```python
from build123d import *

# Parameters (mm, degrees)
SKETCH1_W           = 70
SKETCH1_H           = 70
BOSS_EXTRUDE1_DEPTH = 2
SKETCH2_W           = 50
SKETCH2_H           = 50
BOSS_EXTRUDE2_DEPTH = 35
SKETCH3_R           = 11
CUT_EXTRUDE1_DEPTH  = 6
SKETCH4_R           = 10
CUT_EXTRUDE2_DEPTH  = 2
SKETCH5_W           = 26.5
SKETCH5_H           = 12.5
CUT_EXTRUDE3_DEPTH  = 106.683489723
SKETCH7_W           = 5
SKETCH7_H           = 5.02305645
CUT_EXTRUDE4_DEPTH  = 96.557574268
SKETCH8_W           = 5
SKETCH8_H           = 12.5
CUT_EXTRUDE5_DEPTH  = 18


with BuildPart() as part:
    # Sketch1 → Boss-Extrude1 (new body)
    with BuildSketch(Plane.XY):
        with Locations((35, -35)):
            Rectangle(SKETCH1_W, SKETCH1_H)
    extrude(amount=BOSS_EXTRUDE1_DEPTH)

    # Sketch2 → Boss-Extrude2 (add)
    with BuildSketch(Plane.XY.offset(2)):
        with Locations((35, -35)):
            Rectangle(SKETCH2_W, SKETCH2_H)
    extrude(amount=BOSS_EXTRUDE2_DEPTH)

    # Sketch3 → Cut-Extrude1 (cut)
    with BuildSketch(Plane.XY.offset(37)):
        with Locations((35, -35)):
            Circle(SKETCH3_R)
    extrude(amount=-CUT_EXTRUDE1_DEPTH, mode=Mode.SUBTRACT)

    # Sketch4 → Cut-Extrude2 (cut)
    with BuildSketch(Plane.XY.offset(31)):
        with Locations((35, -35)):
            Circle(SKETCH4_R)
    extrude(amount=-CUT_EXTRUDE2_DEPTH, mode=Mode.SUBTRACT)

    # Sketch5 → Cut-Extrude3 (cut, through all)
    with BuildSketch(Plane.XY.offset(37)):
        with Locations((40.25, -35)):
            Rectangle(SKETCH5_W, SKETCH5_H)
    extrude(amount=-CUT_EXTRUDE3_DEPTH, mode=Mode.SUBTRACT)

    # Sketch7 → Cut-Extrude4 (cut, through all)
    with BuildSketch(Plane.ZY.offset(-53.5)):
        with Locations((2.5, -35)):
            Rectangle(SKETCH7_W, SKETCH7_H)
    extrude(amount=CUT_EXTRUDE4_DEPTH, mode=Mode.SUBTRACT)

    # Sketch8 → Cut-Extrude5 (cut)
    with BuildSketch(Plane.XY.offset(37)):
        with Locations((56, -35)):
            Rectangle(SKETCH8_W, SKETCH8_H)
        with Locations((24.5, -35)):
            Rectangle(SKETCH8_W, SKETCH8_H)
    extrude(amount=-CUT_EXTRUDE5_DEPTH, mode=Mode.SUBTRACT)


solid = part.part
```
Source: CAD feature listing. Evaluate the final solid. Frame: model axes, mm. A direction names the side the tool comes from. Coordinates: 2 decimals unless noted, no trailing zeros. Write each loop counter-clockwise with the first axis right and the second up, starting at its lowest first coordinate (ties: lowest second). Pieces come first, ordered by that corner, then holes. Notation, with made-up numbers: (42, 68) -> (88, 68) arc R22 cw to (88, 74) -> close; hole circle Ø11 at (-22, 9.25). An arc over 180 degrees is marked (long way). Return JSON: item names as keys, results as strings. Group by question number.
1) Section query A-A, the plane y = -35.5. Return loops of the section in (x, z).
2) Section query C-C, the plane x = 11.5. Return loops of the section in (y, z), plus the area to 3 significant figures.
3) Set-up query: faces 1 (the face through (60, -35, 19)), 2 (the face through (35, -60, 19)), 3 (the face through (35, -10, 19)), 4 (the face through (35, -45.2, 31)). Return all of +Z, -Z, +X, -X, +Y, -Y with unobstructed straight access to the full face (end or side cutting, diameter ignored); none if empty.
4) Section query B-B, the plane z = 14. Return loops of the section in (x, y), plus the area to 3 significant figures.
5) Ray query, line 1 along X through (y, z) = (-32, 8); line 2 along Y through (x, z) = (48.5, 3.5); line 3 along X through (y, z) = (-29.5, 28). Return the intervals inside material, ascending.
6) Mould query, pull axis X, two halves, no side actions, for faces 5 (the face through (24, -35, 19)), 6 (the face through (10, -35, 19)), 7 (the face through (66, -35, 2)). Classes: +X half, -X half, draft (parallel to the pull), parting line (faces both ways), or undercut.
7) Section query D-D, the plane y = -56. Return loops of the section in (x, z).
8) Contact query for flat-ended pins moving along their axis: P1, Ø2.5, axis at x = 34, y = -26.5, coming from the +Z side; P2, Ø5.5, axis at x = 56.5, y = -35.5, coming from the +Z side; P3, Ø2, axis at x = 44, z = 8, coming from the +Y side; P4, Ø17.5, axis at y = -30.5, z = 15.5, coming from the -X side. Output: stop coordinate, or through.
From the geometry:
{
 "1": {"outline": "(10, 5) -> (27, 5) -> (27, 19) -> (22, 19) -> (22, 37) -> (10, 37) -> close; (53.5, 0) -> (70, 0) -> (70, 2) -> (60, 2) -> (60, 37) -> (58.5, 37) -> (58.5, 19) -> (53.5, 19) -> close"},
 "2": {"outline": "(-70, 0) -> (-37.51, 0) -> (-37.51, 5) -> (-32.49, 5) -> (-32.49, 0) -> (0, 0) -> (0, 2) -> (-10, 2) -> (-10, 37) -> (-60, 37) -> (-60, 2) -> (-70, 2) -> close", "area": "1,860 mm²"},
 "3": {"face 1": "+Z, +X, +Y, -Y", "face 2": "+Z, +X, -X, -Y", "face 3": "+Z, +X, -X, +Y", "face 4": "+Z"},
 "4": {"outline": "(10, -60) -> (60, -60) -> (60, -10) -> (10, -10) -> close; hole (27, -41.25) -> (53.5, -41.25) -> (53.5, -28.75) -> (27, -28.75) -> close", "area": "2,170 mm²"},
 "5": {"line 1": "10 to 27, 53.5 to 60", "line 2": "-60 to -41.25, -28.75 to -10", "line 3": "10 to 22, 58.5 to 60"},
 "6": {"face 5": "undercut", "face 6": "-X half", "face 7": "draft"},
 "7": {"outline": "(0, 0) -> (70, 0) -> (70, 2) -> (60, 2) -> (60, 37) -> (10, 37) -> (10, 2) -> (0, 2) -> close"},
 "8": {"P1": "z = 29", "P2": "z = 37", "P3": "y = -10", "P4": "x = 10"}
}
